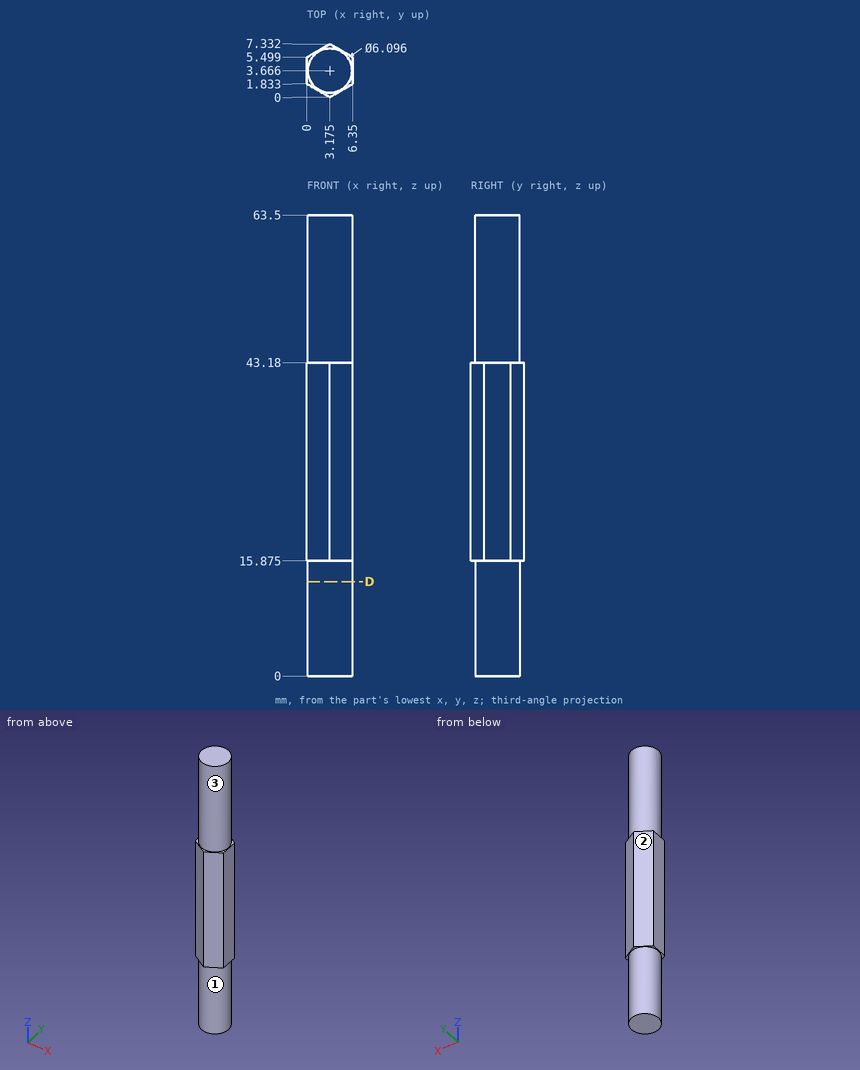
Geometry check sheet. Reference: drawing and pictorial views, mm from the part's lowest x, y, z. A direction names the side the tool comes from. Coordinates: 2 decimals unless noted, no trailing zeros. Order: outer loops, then holes, each group sorted by start corner. A loop starts at its lowest first (then second) coordinate and runs counter-clockwise, first axis right, second up. Notation, with made-up numbers: (-5, 51.5) -> (3, 51.5) arc R32 cw to (3, 85.5) -> close; hole circle Ø9 at (5.25, 1.25). An arc over 180 degrees is marked (long way). Put each result on its own line as item: value. Start each with the question number.
1) Tool access check on the marked faces 1, 2 and 3. Record the directions out of +Z, -Z, +X, -X, +Y, -Y that give a thin tool (end or side, any length) a straight path to the whole face; none if there is none.
2) Cross-section at D-D (z = 13). Enter the section's corners in (x, y) (1 decimal).
3) Material ranges on L1, parallel to Z at x = 0.75, y = 5.75 (1 decimal); L2, parallel to Y at x = 0.5, z = 34 (1 decimal); L3, parallel to X at y = 1.25, z = 59 (1 decimal), recorded low to high.
4) Go/stop test with a flat-tipped pin: pin 1 (1.9 mm diameter, centred on x = 4.5, y = 2.5, fed in from -Z). Record where the tip stops, or that it passes through.
Geometry check:
1. face 1: -Z
1. face 2: +Z, -Z, -X, +Y
1. face 3: +Z
2. outline: circle Ø6.1 at (3.2, 3.7)
3. L1: z = 15.9 to 43.2
3. L2: y = 1.5 to 5.8
3. L3: x = 1.3 to 5
4. pin 1: stops at z = 0
